```python
from build123d import *

# Parameters (mm, degrees)
SKETCH3_W           = 25
SKETCH3_H           = 15
BOSS_EXTRUDE1_DEPTH = 10
CUT_EXTRUDE1_DEPTH  = 2


with BuildPart() as part:
    # Sketch3 → Boss-Extrude1 (new body)
    with BuildSketch(Plane(origin=(0, 0, 0), x_dir=(1, 0, 0), z_dir=(0, 1, 0))):
        with Locations((15.783531292, 6.904865991)):
            Rectangle(SKETCH3_W, SKETCH3_H)
    extrude(amount=BOSS_EXTRUDE1_DEPTH)

    # Sketch4 → Cut-Extrude1 (cut)
    with BuildSketch(Plane.XZ):
        with BuildLine():
            Line((9.428221161, -5.210285602), (13.341179834, -10.757171936))
            Line((13.341179834, -10.757171936), (15.591615362, -13.947318093))
            Line((15.591615362, -13.947318093), (15.938880382, -14.404865991))
            Line((15.938880382, -14.404865991), (14.943009948, -14.404865991))
            Line((14.943009948, -14.404865991), (12.69257442, -11.214719833))
            Line((12.69257442, -11.214719833), (8.779615747, -5.667833499))
            ThreePointArc((8.779615747, -5.667833499), (6.372917751, -3.323604758), (3.283531292, -2.003265808))
            Line((3.283531292, -2.003265808), (3.283531292, -1.189966261))
            Line((3.283531292, -1.189966261), (3.456519377, -1.228595436))
            ThreePointArc((3.456519377, -1.228595436), (6.813253572, -2.6631932), (9.428221161, -5.210285602))
        make_face()
    extrude(amount=-CUT_EXTRUDE1_DEPTH, mode=Mode.SUBTRACT)


solid = part.part
```
Here's how the part is built. I have some questions about the finished solid (model axes, mm). A direction names the side the tool comes from. Give positions to 0.01 mm unless a question says otherwise; leave off trailing zeros. Loops run counter-clockwise (first coordinate to the right, second up) from the corner with the lowest first, then second, coordinate; pieces in that order, holes last. Notation, with made-up numbers: M -16,80 L 0,80 A20 cw 0,89 Z; hole C -9.75,-13 d2. An arc over 180 degrees is marked long. Put each result on its own line as item: value. Start each with the question number.
(1) I want a section at A-A on x = 10.25. Please give me the cut outline in (y, z), then the cut area to 3 significant figures.
(2) I need wall thicknesses on line 1 along Z through (x, y) = (10.25, 1); line 2 along X through (y, z) = (1.75, -3.75); line 3 along X through (y, z) = (1.5, -5.5). Which ranges of each line are inside material? Lowest first, please. Write a range as [from, to].
(3) If we mould it in two halves opening along X, with no side actions, what happens to faces 1 (the flat face through (28.284, 5, -7)), 2 (the flat face through (8, 0, -10)), 3 (the flat face through (10, 2, -7))? For each: +X half, -X half, draft (parallel to the pull), parting line (faces both ways), or undercut.
(4) For faces 4 (the flat face through (16, 10, -7)), 5 (the cylindrical face through (6.41, 0.99, -3.35)), which set-ups out of +Z, -Z, +X, -X, +Y, -Y let a thin tool reach every point of the face, with its end or its side?
Answer block:
1. outline: M 0,-14.4 L 10,-14.4 L 10,0.6 L 0,0.6 L 0,-6.38 L 2,-6.38 L 2,-7.75 L 0,-7.75 Z
1. area: 147 mm^2
2. line 1: [-14.4, -7.75], [-6.38, 0.6]
2. line 2: [3.28, 6.96], [8.17, 28.28]
2. line 3: [3.28, 8.66], [9.63, 28.28]
3. face 1: +X half
3. face 2: draft
3. face 3: undercut
4. face 4: +Z, -Z, +X, -X, +Y
4. face 5: -Y
